Check sheet for the drawn part. Datum: minimum x, y, z corner. Units: mm. A direction names the side the tool comes from. Round coordinates to 2 decimals unless told otherwise and drop trailing zeros. Write each loop counter-clockwise with the first axis right and the second up, starting at its lowest first coordinate (ties: lowest second). Pieces come first, ordered by that corner, then holes. Notation, with made-up numbers: M 69,-1.75 L 77,-1.75 A7 ccw 77,5.25 Z; hole C 18,66.5 d3. An arc over 180 degrees is marked long. One line per item, written item: value. Start each with the question number.
1. Section check B-B (x = 12.7). Record the boundary of the cut face in (y, z) (1 decimal), and give its area (3 significant figures).
2. Section check D-D (y = 4.75). Record the boundary of the cut face in (x, z), and give its area (3 significant figures).
3. Section check A-A (x = 8.25). Record the boundary of the cut face in (y, z) (1 decimal).
4. Scan lines: probe 1 along Z at (x, y) = (11.5, 14); probe 2 along Z at (x, y) = (9.5, 17.75); probe 3 along Y at (x, z) = (13, 30). Record each from-to range of solid material in increasing order. Write a range as [from, to].
5. Section check C-C (z = 49). Record the boundary of the cut face in (x, y), and give its area (3 significant figures).
6. Depth check by flat-ended pin: P1, Ø3.5, axis at y = 12.7, z = 73.99, coming from the -X side; P2, Ø3, axis at x = 16.5, z = 63.5, coming from the +Y side (1 decimal); P3, Ø1.5, axis at x = 14.5, y = 21, coming from the +Z side; P4, Ø2.5, axis at y = 12.7, z = 73.99, coming from the +X side. Enter the tip coordinate at first touch or a pass-through.
7. Access from +Z, -Z, +X, -X, +Y, -Y to the whole of each face (thin tool, end or side, straight path). Record for the marked faces 1 and 2.
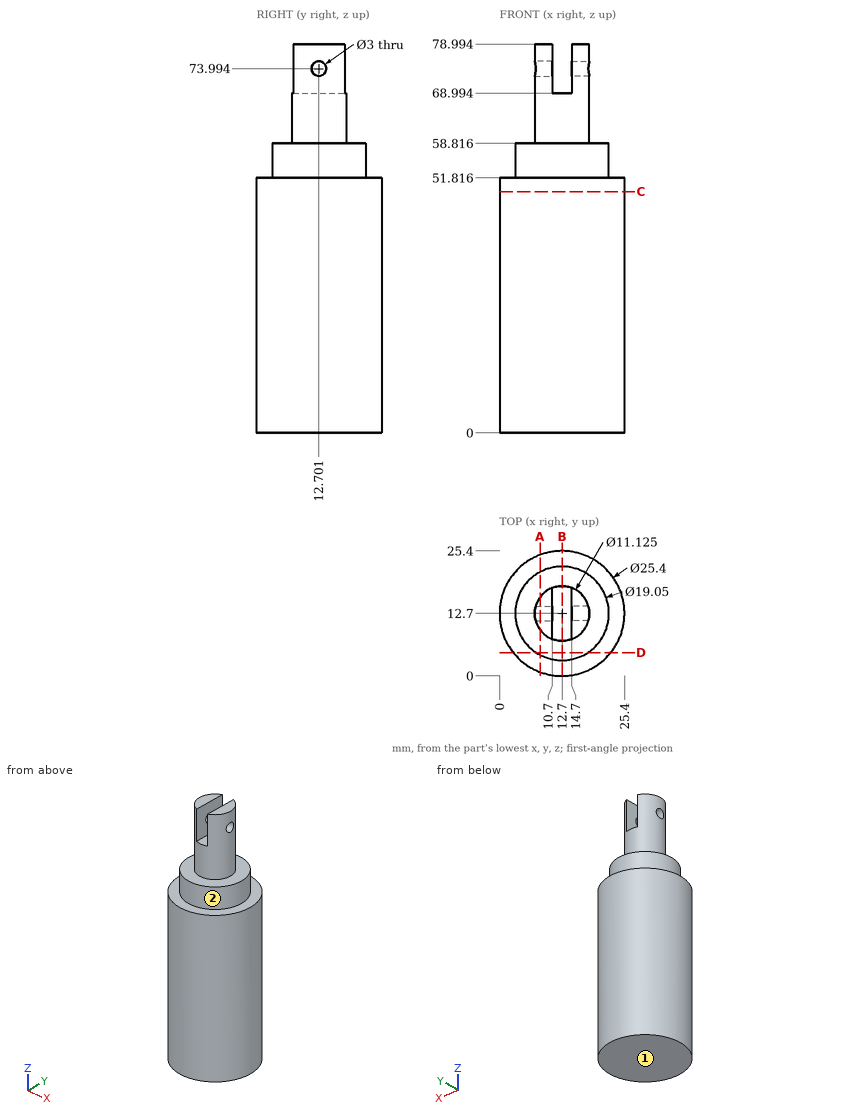
Result sheet:
1. outline: M 0,0 L 25.4,0 L 25.4,51.8 L 22.2,51.8 L 22.2,58.8 L 18.3,58.8 L 18.3,69 L 7.1,69 L 7.1,58.8 L 3.2,58.8 L 3.2,51.8 L 0,51.8 Z
1. area: 1,560 mm2
2. outline: M 2.8,0 L 22.6,0 L 22.6,51.82 L 17.95,51.82 L 17.95,58.82 L 7.45,58.82 L 7.45,51.82 L 2.8,51.82 Z
2. area: 1,100 mm2
3. outline: M 0.8,0 L 24.6,0 L 24.6,51.8 L 21.1,51.8 L 21.1,58.8 L 16,58.8 L 16,79 L 9.4,79 L 9.4,58.8 L 4.3,58.8 L 4.3,51.8 L 0.8,51.8 Z; hole C 12.7,74 d3
4. probe 1: z = [0, 68.99]
4. probe 2: z = [0, 58.82]
4. probe 3: y = [0, 25.4]
5. outline: C 12.7,12.7 d25.4
5. area: 507 mm2
6. P1: stops at x = 7.14
6. P2: stops at y = 17.8
6. P3: stops at z = 58.82
6. P4: passes through
7. face 1: -Z, +X, -X, +Y, -Y
7. face 2: +Z
